Work out the finished part from the listing and answer in its coordinate system (mm). A direction names the side the tool comes from. Coordinates: 2 decimals unless noted, no trailing zeros. Write each loop counter-clockwise with the first axis right and the second up, starting at its lowest first coordinate (ties: lowest second). Pieces come first, ordered by that corner, then holes. Notation, with made-up numbers: (24.5, -21.5) - (69.5, -21.5) arc R3 ccw to (69.5, -17.5) - close; hole circle Ø10 at (-20, 26.5). An arc over 180 degrees is marked (long way). Answer as a JSON object with one key per item and string values. Group by question number.
from build123d import *

# Parameters (mm, degrees)
F0_W     = 60
F0_H     = 60
F1_DEPTH = 25
F2_R     = 5
F3_DEPTH = 25


with BuildPart() as f1:
    # F0 (on Top) → F1 (new body)
    with BuildSketch(Plane.XY):
        Rectangle(F0_W, F0_H)
    extrude(amount=F1_DEPTH)

    # F2 (on face) → F3 (join)
    with BuildSketch(Plane.YZ.offset(30)):
        with Locations((15, 5)):
            Circle(F2_R)
    extrude(amount=F3_DEPTH)


solid = f1.part
Q1. Section C-C on x = 38 is taken. Determine the outline of the cut face in (y, z).
Q2. Flat-ended cylindrical pins translate along their axes: pin 1 Ø4 at (x, y) = (41, 20) entering from +Z; pin 2 Ø2 at (y, z) = (23, 6) entering from +X. Find the tip coordinate at first contact, or state that the pin passes through.
Q3. Section A-A on z = 5 is taken. Determine the outline of the cut face in (x, y).
Q4. Section D-D on z = 22.75 is taken. Determine the outline of the cut face in (x, y).
Q5. Section B-B on y = -9.5 is taken. Determine the outline of the cut face in (x, z).
Q6. Consider L1, parallel to X at y = 8.5, z = 12.75; L2, parallel to Y at x = 38.5, z = 4.5. Determine where each line is inside the solid, lowest interval first. Write a range as from..to.
Q7. A tool of negligible diameter and unlimited length cuts with its end or side. For faces 1 (the face through (55, 15, 5)), 2 (the face through (42.325, 19.619, 3.085)), from which of +Z, -Z, +X, -X, +Y, -Y can it reach the whole face along a straight path? Write none if from no direction.
Numbers:
{
 "1": {"outline": "circle Ø10 at (15, 5)"},
 "2": {"pin 1": "stops at z = 9", "pin 2": "stops at x = 30"},
 "3": {"outline": "(-30, -30) - (30, -30) - (30, 10) - (55, 10) - (55, 20) - (30, 20) - (30, 30) - (-30, 30) - close"},
 "4": {"outline": "(-30, -30) - (30, -30) - (30, 30) - (-30, 30) - close"},
 "5": {"outline": "(-30, 0) - (30, 0) - (30, 25) - (-30, 25) - close"},
 "6": {"L1": "x = -30..30", "L2": "y = 10.03..19.97"},
 "7": {"face 1": "+Z, -Z, +X, +Y, -Y", "face 2": "+X"}
}
